```python
from build123d import *

# Parameters (mm, degrees)
F0_W     = 60
F0_H     = 104
F1_DEPTH = 40
F3_D     = 26
F3_DEPTH = 104
F3_TIP   = 7.8111880474
F5_D     = 11
F5_DEPTH = 104
F5_TIP   = 3.3047334047


with BuildPart() as f1:
    # F0 (on Front) → F1 (new body)
    with BuildSketch(Plane.XZ):
        Rectangle(F0_W, F0_H)
    extrude(amount=F1_DEPTH)

    # F3
    with Locations(Plane.XY.offset(52)):
        with Locations((0, -20)):
            Hole(F3_D / 2, depth=F3_DEPTH)
            with Locations((0, 0, -(F3_DEPTH + F3_TIP / 2))):  # 118° drill point
                Cone(0, F3_D / 2, F3_TIP, mode=Mode.SUBTRACT)

    # F5
    with Locations(Plane.XZ.offset(40)):
        with Locations((-20, 20), (-20, -20), (20, -20), (20, 20)):
            Hole(F5_D / 2, depth=F5_DEPTH)
            with Locations((0, 0, -(F5_DEPTH + F5_TIP / 2))):  # 118° drill point
                Cone(0, F5_D / 2, F5_TIP, mode=Mode.SUBTRACT)


solid = f1.part
```
Can you work these out from the model? Positions are in its coordinate system, mm. Give positions to 0.01 mm unless a question says otherwise; leave off trailing zeros. Loops run counter-clockwise (first coordinate to the right, second up) from the corner with the lowest first, then second, coordinate; pieces in that order, holes last. Notation, with made-up numbers: M 85.5,54.25 L 136.5,54.25 A23 cw 136.5,63.25 Z; hole C 60.5,69 d10. An arc over 180 degrees is marked long. One line per item, written item: value.
(1) Suppose I cut it at B-B on z = 20. List the corners of the cut face in (x, y) for me.
Returned:
outline: M -30,-40 L -25.5,-40 L -25.5,0 L -30,0 Z; M -14.5,-40 L 14.5,-40 L 14.5,0 L -14.5,0 Z; M 25.5,-40 L 30,-40 L 30,0 L 25.5,0 Z; hole C 0,-20 d26
(2) Suppose I cut it at D-D on y = -5. List the corners of the cut face in (x, z) for me, plus the area to 3 significant figures.
Returned:
outline: M -30,-52 L 30,-52 L 30,52 L -30,52 Z; hole C -20,-20 d11; hole C -20,20 d11; hole C 20,-20 d11; hole C 20,20 d11
area: 5,860 mm^2
(3) Suppose I cut it at A-A on y = -20. List the corners of the cut face in (x, z) for me, plus the area to 3 significant figures.
Returned:
outline: M -30,-52 L -13,-52 L -13,52 L -30,52 Z; M 13,-52 L 30,-52 L 30,52 L 13,52 Z; hole C -20,-20 d11; hole C -20,20 d11; hole C 20,-20 d11; hole C 20,20 d11
area: 3,160 mm^2
(4) We'd pull the mould along X, two halves only. Please class faces 1 (the face through (30, -20, -1)), 2 (the face through (14.92, -19.72, -22.11)), 3 (the face through (0, -40, 1)), 4 (the face through (-30, -20, -1)): released by +X, released by -X, zero draft, split by the parting line, or undercut.
Returned:
face 1: released by +X
face 2: undercut
face 3: zero draft
face 4: released by -X
(5) Suppose I cut it at C-C on x = 20. List the corners of the cut face in (y, z) for me.
Returned:
outline: M -40,-52 L 0,-52 L 0,-25.5 L -40,-25.5 Z; M -40,-14.5 L 0,-14.5 L 0,14.5 L -40,14.5 Z; M -40,25.5 L 0,25.5 L 0,52 L -40,52 Z
(6) I need wall thicknesses on line 1 (Z direction, x = -20.5, y = -8.5); line 2 (X direction, y = -20, z = 3); line 3 (Y direction, x = 0, z = -19.5). Which ranges of each line are inside material? Lowest first, please.
Returned:
line 1: -52 to -25.48, -14.52 to 14.52, 25.48 to 52
line 2: -30 to -13, 13 to 30
line 3: -40 to -33, -7 to 0
(7) Will this pin go through, and if not, where does the flat tip stop? pin 1 (10 mm diameter, centred on x = -20, z = 20, fed in from -Y).
Returned:
pin 1: through
